Part model, mm, in its own coordinate system. Face numbers are marked on the shaded views. A direction names the side the tool comes from. Round coordinates to 2 decimals unless told otherwise and drop trailing zeros. Loops run counter-clockwise (first coordinate to the right, second up) from the corner with the lowest first, then second, coordinate; pieces in that order, holes last. Notation, with made-up numbers: (-34.75, 63) -> (16.25, 63) arc R15 ccw to (16.25, 88) -> close; hole circle Ø5 at (57, 81). An arc over 180 degrees is marked (long way). Use a Markdown table: item, result. Add a question column.
Item 1: Cut at A-A, the plane x = 1. List the corners of the cut face in (y, z).
Item 2: Cut at C-C, the plane z = -8.25. List the corners of the cut face in (x, y), plus the area to 3 significant figures.
Item 3: Cut at B-B, the plane y = 1. List the corners of the cut face in (x, z).
Item 4: Which spindle directions (+Z, -Z, +X, -X, +Y, -Y) get a long thin tool onto all of the face, cutting with end or side? Do the marked faces 4 and 5. Say none if no direction does.
Item 5: Flat gauge pins, fed straight in: pin 1 (1.5 mm diameter, centred on x = 2, z = -10.5, fed in from +Y); pin 2 (4 mm diameter, centred on x = 0, y = 0, fed in from -Z); pin 3 (10 mm diameter, centred on x = 8.5, z = -3.5, fed in from -Y); pin 4 (2 mm diameter, centred on x = -3.5, z = -8, fed in from -Y). Where does each tip first touch, or does it go through?
Item 6: Probe line 1 (Z direction, x = -2, y = -33.5); line 2 (Y direction, x = 0, z = -13.25); line 3 (X direction, y = 0, z = 1.25). List the from-to ranges inside material, lowest first. Write a range as [from, to].
Item 7: Cut at D-D, the plane x = -4. List the corners of the cut face in (y, z).
Item 8: Two-plate mould, pull along Y, no slides. Class the marked faces 1, 2 and 3: pulls with the +Y half, pulls with the -Y half, needs draft (parallel to the pull), parting line crosses it, or undercut.
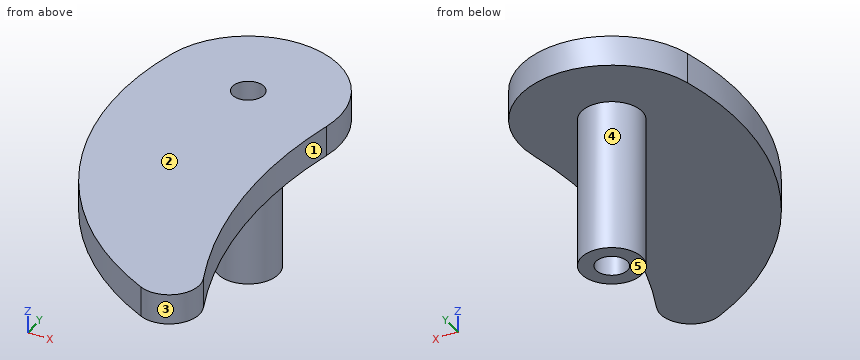
Autodesk Inventor part; units mm, degrees
ref_plane "YZ Plane" through (0, 0, 0) normal (1, 0, 0) x (0, 1, 0)
ref_plane "XZ Plane" through (0, 0, 0) normal (0, 1, 0) x (-1, 0, 0)
ref_plane "XY Plane" through (0, 0, 0) normal (0, 0, 1) x (1, 0, 0)
sketch "Sketch1" plane through (0, 0, 0) normal (0, 0, 1) x (1, 0, 0)
  circle A0 centre (0, 0) radius 15
  circle A1 centre (15, -50) radius 5
  arc A2 (14.7146, -2.9124) -> (19.5845, -48.0044) centre (89.2722, -17.6691) ccw
  arc A3 (-14.5962, 3.4571) -> (12.8032, -54.4915) centre (35.3589, -8.3749) ccw
  point P0 (15, -55)
  point P1 (13.6233, -6.2774)
  point P2 (15, -45)
  dimension "d0" = 30
  dimension "d1" = 10
  dimension "d2" = 15
  dimension "d3" = 50
extrude "Extrusion1" add sketch "Sketch1" along normal blind 5
sketch "Sketch2" plane through (0, 0, 5) normal (0, 0, 1) x (1, 0, 0)
  circle A0 centre (0, 0) radius 2.6
  dimension "d8" = 5.2
extrude "Extrusion2" cut sketch "Sketch2" against normal blind 40
sketch "Sketch3" plane through (0, 0, 0) normal (0, 0, -1) x (-1, 0, 0)
  circle A0 centre (0, 0) radius 2.6
  circle A1 centre (0, 0) radius 5
  circle A2 centre (0, 0) radius 2.6
  dimension "d13" = 10
extrude "Extrusion3" add sketch "Sketch3" along normal blind 25
properties part number "p2_3DPrint"
A:
| question | item | result |
|---|---|---|
| 1 | outline | (-46.52, 0) -> (-4.9, 0) -> (-4.9, -25) -> (-2.4, -25) -> (-2.4, 5) -> (-46.52, 5) -> close; (2.4, -25) -> (4.9, -25) -> (4.9, 0) -> (14.97, 0) -> (14.97, 5) -> (2.4, 5) -> close |
| 2 | outline | circle Ø10 at (0, 0); hole circle Ø5.2 at (0, 0) |
| 2 | area | 57.3 mm^2 |
| 3 | outline | (-15.12, 0) -> (-4.9, 0) -> (-4.9, -25) -> (-2.4, -25) -> (-2.4, 5) -> (-15.12, 5) -> close; (2.4, -25) -> (4.9, -25) -> (4.9, 0) -> (14.97, 0) -> (14.97, 5) -> (2.4, 5) -> close |
| 4 | face 4 | -Z |
| 4 | face 5 | -Z, +X, -X, +Y, -Y |
| 5 | pin 1 | stops at y = 4.84 |
| 5 | pin 2 | passes through |
| 5 | pin 3 | stops at y = -54.13 |
| 5 | pin 4 | stops at y = -4.33 |
| 6 | line 1 | z = [0, 5] |
| 6 | line 2 | y = [-5, -2.6], [2.6, 5] |
| 6 | line 3 | x = [-15.29, -2.6], [2.6, 15] |
| 7 | outline | (-41.34, 0) -> (-3, 0) -> (-3, -25) -> (3, -25) -> (3, 0) -> (14.46, 0) -> (14.46, 5) -> (-41.34, 5) -> close |
| 8 | face 1 | undercut |
| 8 | face 2 | needs draft |
| 8 | face 3 | parting line crosses it |
